from build123d import *

# Parameters (mm, degrees)
F0_W      = 26.5
F0_H      = 35
F1_DEPTH  = 16.5
F2_W      = 20.5
F2_H      = 10.5
F3_DEPTH  = 35
F4_W      = 6
F4_H      = 20
F5_DEPTH  = 30
F7_DEPTH  = 20
F8_R      = 3.75
F9_DEPTH  = 25
F10_W     = 3.944425
F10_H     = 8.5
F11_DEPTH = 25
F12_R     = 2.7
F12_R_2   = 1.65
F13_DEPTH = 2


with BuildPart() as f1:
    # F0 (on Front) → F1 (new body)
    with BuildSketch(Plane.XZ):
        Rectangle(F0_W, F0_H)
    extrude(amount=F1_DEPTH)

    # F2 (on face) → F3 (cut)
    with BuildSketch(Plane.XY.offset(17.5)):
        with Locations((0, -8.25)):
            Rectangle(F2_W, F2_H)
    extrude(amount=-F3_DEPTH, mode=Mode.SUBTRACT)

    # F4 (on face) → F5 (join)
    with BuildSketch(Plane.YZ.offset(13.25)):
        with Locations((-13.5, 0.5)):
            Rectangle(F4_W, F4_H)
    extrude(amount=F5_DEPTH)

    # F6 (on face) → F7 (join)
    with BuildSketch(Plane(origin=(0, 0, -9.5), x_dir=(1, 0, 0), z_dir=(0, 0, -1))):
        Polygon((13.25, 5.5), (17.25, 10.5), (13.25, 10.5), align=None)
    extrude(amount=-F7_DEPTH)

    # F8 (on face) → F9 (cut)
    with BuildSketch(Plane.XZ.offset(16.5)):
        with Locations((28.25, 0)):
            Circle(F8_R)
    extrude(amount=-F9_DEPTH, mode=Mode.SUBTRACT)

    # F10 (on face) → F11 (cut)
    with BuildSketch(Plane(origin=(0, -10.5, 0), x_dir=(-1, 0, 0), z_dir=(0, 1, 0))):
        with Locations((-15.277787, 0.005)):
            Rectangle(F10_W, F10_H)
    extrude(amount=F11_DEPTH, mode=Mode.SUBTRACT)

    # F12 (on face) → F13 (join)
    with BuildSketch(Plane(origin=(0, 0, 0), x_dir=(-1, 0, 0), z_dir=(0, 1, 0))):
        Circle(F12_R)
        Circle(F12_R_2, mode=Mode.SUBTRACT)
        with Locations((0, 9.5)):
            Circle(F12_R)
        with Locations((0, 9.5)):
            Circle(F12_R_2, mode=Mode.SUBTRACT)
        with Locations((0, -11)):
            Circle(F12_R)
        with Locations((0, -11)):
            Circle(F12_R_2, mode=Mode.SUBTRACT)
    extrude(amount=F13_DEPTH)


solid = f1.part
Part model, mm, in its own coordinate system. A direction names the side the tool comes from. Coordinates: 2 decimals unless noted, no trailing zeros. Loops run counter-clockwise (first coordinate to the right, second up) from the corner with the lowest first, then second, coordinate; pieces in that order, holes last. Notation, with made-up numbers: M -16,32 L 27,32 A15 cw 27,37 Z; hole C 1,14 d4. An arc over 180 degrees is marked long. Use a Markdown table: item, result. Add a question column.
Q1. Probe L1, parallel to Z at x = 0, y = 0.8; L2, parallel to Y at x = 2, z = -13; L3, parallel to X at y = -5.75, z = -2. List the from-to ranges inside material, lowest first.
Q2. Mould opens along X. For faces 1 (the flat face through (0, 2, -2)), 2 (the flat face through (-10.25, -8, 0)), 3 (the flat face through (15.22, -7.96, 4.8)) say: +X half, -X half, draft (parallel to the pull), parting line (faces both ways), or undercut.
Q3. Pin check, flat tips, straight feed: P1, Ø4.5, axis at x = 16, y = -7.5, coming from the -Z side; P2, Ø1, axis at x = 15.5, z = -9.5, coming from the +Y side; P3, Ø1.5, axis at y = -7.5, z = 6, coming from the +X side. Stop position of each tip, or through.
Q4. Cut at A-A (x = -9). Write the cut outline in (y, z).
Q5. Cut at C-C (y = -14.25). Write the cut outline in (x, z).
Q6. Which spindle directions (+Z, -Z, +X, -X, +Y, -Y) get a long thin tool onto all of the face, cutting with end or side? Do faces 4 (the flat face through (15, -9, 4.255)), 5 (the flat face through (-13.25, -8, 0)), 6 (the flat face through (28, -14, -9.5)), 7 (the cylindrical face through (0.585, 0.986, -2.636)). Say none if no direction does.
Q7. Cut at B-B (z = -11). Write the cut outline in (x, y), and give its area (3 significant figures).
Worked out:
| question | item | result |
|---|---|---|
| 1 | L1 | z = -13.7 to -12.65, -9.35 to -8.3, -2.7 to -1.65, 1.65 to 2.7, 6.8 to 7.85, 11.15 to 12.2 |
| 1 | L2 | y = -16.5 to -13.5, -3 to 0 |
| 1 | L3 | x = -13.25 to -10.25, 10.25 to 13.31 |
| 2 | face 1 | draft |
| 2 | face 2 | undercut |
| 2 | face 3 | +X half |
| 3 | P1 | stops at z = -9.5 |
| 3 | P2 | stops at y = -7.69 |
| 3 | P3 | stops at x = 15.45 |
| 4 | outline | M -16.5,-17.5 L -13.5,-17.5 L -13.5,17.5 L -16.5,17.5 Z; M -3,-17.5 L 0,-17.5 L 0,17.5 L -3,17.5 Z |
| 5 | outline | M -13.25,-17.5 L 13.25,-17.5 L 13.25,-9.5 L 43.25,-9.5 L 43.25,10.5 L 13.25,10.5 L 13.25,17.5 L -13.25,17.5 Z; hole C 28.25,0 d7.5 |
| 6 | face 4 | +X, +Y |
| 6 | face 5 | +Z, -Z, -X, +Y, -Y |
| 6 | face 6 | -Z, +X, +Y, -Y |
| 6 | face 7 | +Y |
| 7 | outline | M -13.25,-16.5 L 13.25,-16.5 L 13.25,0 L 2.7,0 L 2.7,2 L 1.65,2 L 1.65,0 L -1.65,0 L -1.65,2 L -2.7,2 L -2.7,0 L -13.25,0 Z; hole M -10.25,-13.5 L 10.25,-13.5 L 10.25,-3 L -10.25,-3 Z |
| 7 | area | 226 mm2 |
